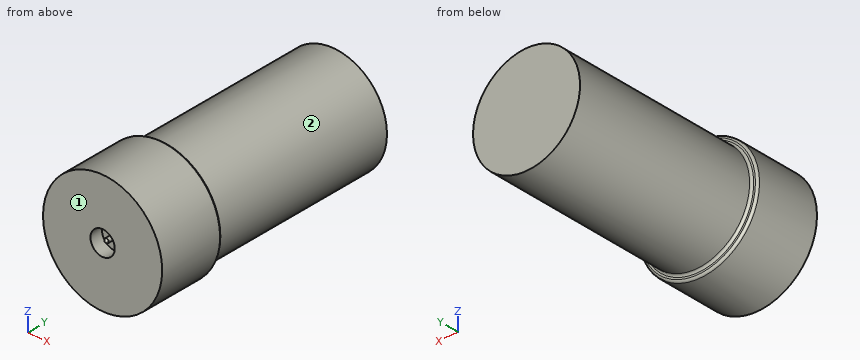
from build123d import *

# Parameters (mm, degrees)
SKETCH1_R           = 13.75
BOSS_EXTRUDE1_DEPTH = 15.35
SKETCH2_R           = 12.35
BOSS_EXTRUDE2_DEPTH = 44.35
FILLET1_R           = 0.5
SKETCH3_R           = 2.8
CUT_EXTRUDE1_DEPTH  = 3
SKETCH4_R           = 0.5
BOSS_EXTRUDE3_DEPTH = 2.5
CHAMFER1_SIZE       = 0.5


with BuildPart() as part:
    # Sketch1 → Boss-Extrude1 (new body)
    with BuildSketch(Plane(origin=(0, 0, 0), x_dir=(1, 0, 0), z_dir=(0, 1, 0))):
        Circle(SKETCH1_R)
    extrude(amount=BOSS_EXTRUDE1_DEPTH)

    # Sketch2 → Boss-Extrude2 (add)
    with BuildSketch(Plane(origin=(0, 15.35, 0), x_dir=(1, 0, 0), z_dir=(0, 1, 0))):
        Circle(SKETCH2_R)
    extrude(amount=BOSS_EXTRUDE2_DEPTH)

    # Fillet1
    fillet1_edges = [part.edges().sort_by_distance(p)[0] for p in [
        (-13.75, 15.35, 0),
        (-12.35, 15.35, 0),
    ]]
    fillet(fillet1_edges, radius=FILLET1_R)

    # Sketch3 → Cut-Extrude1 (cut)
    with BuildSketch(Plane.XZ):
        Circle(SKETCH3_R)
    extrude(amount=-CUT_EXTRUDE1_DEPTH, mode=Mode.SUBTRACT)

    # Sketch4 → Boss-Extrude3 (add)
    with BuildSketch(Plane.XZ.offset(-3)):
        Circle(SKETCH4_R)
    extrude(amount=BOSS_EXTRUDE3_DEPTH)

    # Chamfer1
    chamfer1_edges = [part.edges().sort_by_distance(p)[0] for p in [
        (-0.5, 0.5, 0),
    ]]
    chamfer(chamfer1_edges, length=CHAMFER1_SIZE)


solid = part.part
Design review of the part built by this model. Coordinates are the model's own, in mm. Face numbers are marked on the shaded views. A direction names the side the tool comes from. Round coordinates to 2 decimals unless told otherwise and drop trailing zeros. Order: outer loops, then holes, each group sorted by start corner. A loop starts at its lowest first (then second) coordinate and runs counter-clockwise, first axis right, second up. Notation, with made-up numbers: M -23,1 L 33,1 A24 cw 33,32 Z; hole C -23,30.25 d3. An arc over 180 degrees is marked long. Answer as CSV lines item,"result". Start each with the question number.
1) Wall thickness on line 1 along Z through (x, y) = (0, 1.55); line 2 along Y through (x, z) = (11, 6.5); line 3 along Z through (x, y) = (0, 0.8): over which ranges is each line inside the solid? List them lowest first. Write a range as [from, to].
2) Tool access review of the marked faces 1 and 2: name each direction out of +Z, -Z, +X, -X, +Y, -Y from which nothing blocks a thin tool from reaching the whole face with its end or side.
3) Add section A-A (y = 27.5). Give the boundary of the cut face in (x, z).
4) Add section B-B (y = 5). Give the boundary of the cut face in (x, z), then the cut area to 3 significant figures.
5) For pin 1 Ø6 at (y, z) = (38.5, -4.5) entering from +X; pin 2 Ø10 at (y, z) = (34.5, -8.5) entering from -X; pin 3 Ø3 at (y, z) = (28.5, -11) entering from +X, all flat-tipped, find the tip position at first contact; note any pin that passes through.
Resolved:
1,line 1,"[-13.75, -2.8], [-0.5, 0.5], [2.8, 13.75]"
1,line 2,"[0, 15.36]"
1,line 3,"[-13.75, -2.8], [-0.3, 0.3], [2.8, 13.75]"
2,face 1,"+Z, -Z, +X, -X, -Y"
2,face 2,"+Y"
3,outline,"C 0,0 d24.7"
4,outline,"C 0,0 d27.5"
4,area,"594 mm^2"
5,pin 1,"x = 12.26"
5,pin 2,"x = -11.84"
5,pin 3,"x = 7.89"
